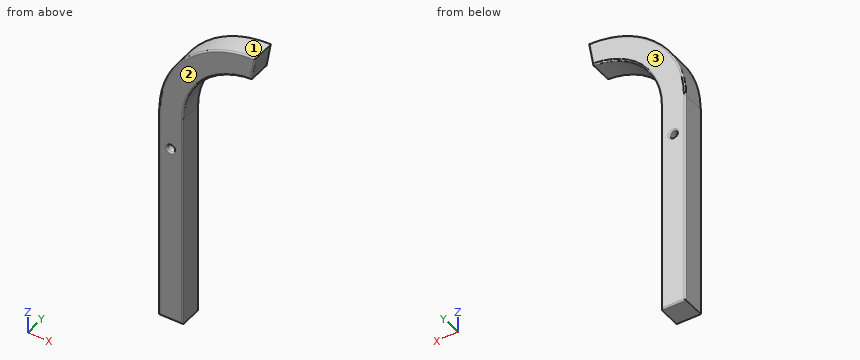
from build123d import *

# Parameters (mm, degrees)
F0_R     = 3.96875
F1_DEPTH = 25.4
F2_R     = 1.524


with BuildPart() as f1:
    # F0 (on Front) → F1 (new body)
    with BuildSketch(Plane.XZ):
        with BuildLine():
            Line((0, 228.6), (0, 0))
            Line((0, 0), (25.4, 0))
            Line((25.4, 0), (25.4, 228.6))
            ThreePointArc((25.4, 228.6), (46.149545, 280.865543), (97.097822, 304.666881))
            Line((97.097822, 304.666881), (101.6, 330.2))
            ThreePointArc((101.6, 330.2), (29.757951, 300.442049), (0, 228.6))
        make_face()
        with Locations((12.7, 190.5)):
            Circle(F0_R, mode=Mode.SUBTRACT)
    extrude(amount=F1_DEPTH)

    # F2
    f2_edges = [f1.edges().sort_by_distance(p)[0] for p in [
        (0, -25.4, 114.3),
        (12.7, -25.4, 0),
        (25.4, -25.4, 114.3),
        (46.149545, -25.4, 280.865543),
        (99.348911, -25.4, 317.433441),
        (29.757951, -25.4, 300.442049),
        (8.73125, -25.4, 190.5),
        (0, 0, 114.3),
        (12.7, 0, 0),
        (25.4, 0, 114.3),
        (46.149545, 0, 280.865543),
        (99.348911, 0, 317.433441),
        (29.757951, 0, 300.442049),
        (8.73125, 0, 190.5),
    ]]
    fillet(f2_edges, radius=F2_R)


solid = f1.part
Could you check a few things on this model? Use its own coordinates, in mm. Face numbers are marked on the shaded views. Round coordinates to 2 decimals unless told otherwise and drop trailing zeros. Write each loop counter-clockwise with the first axis right and the second up, starting at its lowest first coordinate (ties: lowest second). Pieces come first, ordered by that corner, then holes. Notation, with made-up numbers: (-40, -23.75) - (-22, -23.75) arc R20 cw to (-22, 3.25) - close; hole circle Ø10 at (-33, 6). An arc over 180 degrees is marked (long way). Put each result on its own line as item: value. Start each with the question number.
(1) I want a section at C-C, the plane y = -19.5. Please give me the cut outline in (x, z).
(2) I want a section at B-B, the plane z = 155.5. Please give me the cut outline in (x, y), plus the area to 3 significant figures.
(3) I want a section at A-A, the plane z = 190.5. Please give me the cut outline in (x, y).
(4) I need wall thicknesses on probe 1 along X at (y, z) = (-6.5, 124); probe 2 along Z at (x, y) = (12.7, -19.25); probe 3 along Z at (x, y) = (50, -3.75). Which ranges of each line are inside material? Lowest first, please.
(5) Will these pins go through, and if not, where does the flat tip stop? pin 1 (10 mm diameter, centred on y = -10.5, z = 255.5, fed in from +X); pin 2 (10 mm diameter, centred on x = 85.5, z = 295.5, fed in from +Y); pin 3 (2 mm diameter, centred on x = 60, y = -17.5, fed in from -Z); pin 4 (1.5 mm diameter, centred on x = 59.5, y = -19, fed in from +Z).
(6) Thinking about a two-plate mould opening in Y: for the marked faces 1, 2 and 3, which applies, released by +Y, released by -Y, zero draft, split by the parting line, or undercut?
Here are the results:
1. outline: (0, 0) - (25.4, 0) - (25.4, 228.6) arc R76.2 cw to (97.1, 304.67) - (101.6, 330.2) arc R101.6 ccw to (0, 228.6) - close; hole circle Ø7.94 at (12.7, 190.5)
2. outline: (0, -23.88) arc R1.52 ccw to (1.52, -25.4) - (23.88, -25.4) arc R1.52 ccw to (25.4, -23.88) - (25.4, -1.52) arc R1.52 ccw to (23.88, 0) - (1.52, 0) arc R1.52 ccw to (0, -1.52) - close
2. area: 643 mm^2
3. outline: (0, -23.88) arc R1.52 ccw to (1.52, -25.4) - (7.21, -25.4) arc R1.52 ccw to (8.73, -23.88) - (8.73, -1.52) arc R1.52 ccw to (7.21, 0) - (1.52, 0) arc R1.52 ccw to (0, -1.52) - close; (16.67, -23.88) arc R1.52 ccw to (18.19, -25.4) - (23.88, -25.4) arc R1.52 ccw to (25.4, -23.88) - (25.4, -1.52) arc R1.52 ccw to (23.88, 0) - (18.19, 0) arc R1.52 ccw to (16.67, -1.52) - close
4. probe 1: x = 0 to 25.4
4. probe 2: z = 0 to 186.53, 194.47 to 277.79
4. probe 3: z = 284.67 to 316.12
5. pin 1: stops at x = 32.4
5. pin 2: passes through
5. pin 3: stops at z = 291.78
5. pin 4: stops at z = 321.4
6. face 1: zero draft
6. face 2: released by -Y
6. face 3: released by +Y
